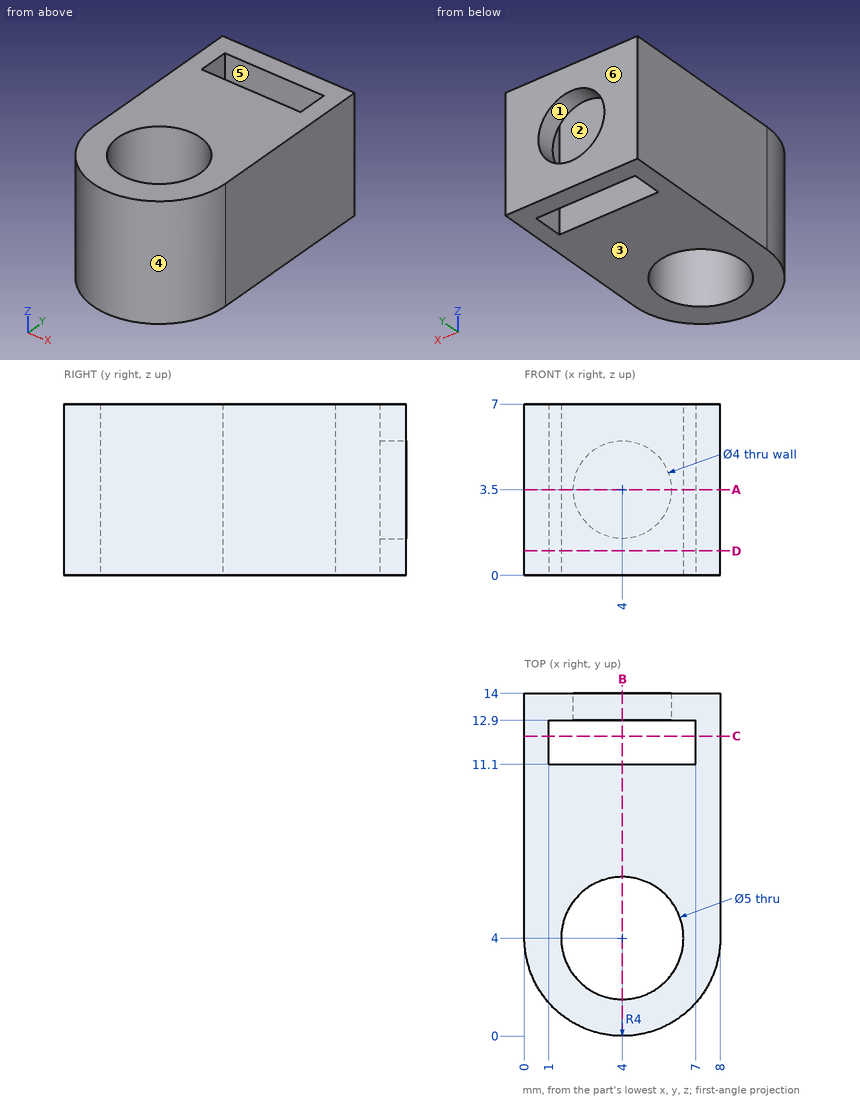
Verification items for this drawing (mm, ordinates from the low corner). A direction names the side the tool comes from. Round coordinates to 2 decimals unless told otherwise and drop trailing zeros. Order: outer loops, then holes, each group sorted by start corner. A loop starts at its lowest first (then second) coordinate and runs counter-clockwise, first axis right, second up. Notation, with made-up numbers: (-1.5, -19) - (10.5, -19) arc R19 cw to (10.5, 9) - close; hole circle Ø9 at (-26.5, -21.5). An arc over 180 degrees is marked (long way). Use CSV: the item, a comma, the result in double quotes. Start each with the question number.
1) Section check B-B, the plane x = 4. Record the cut outline in (y, z), plus the area to 3 significant figures.
2) Go/stop test with a flat-tipped pin: P1, Ø4.5, axis at x = 4, y = 4, coming from the +Z side. Record where the tip stops, or that it passes through.
3) Access from +Z, -Z, +X, -X, +Y, -Y to the whole of each face (thin tool, end or side, straight path). Record for the marked faces 1, 2 and 3.
4) Section check D-D, the plane z = 1. Record the cut outline in (x, y), plus the area to 3 significant figures.
5) Section check A-A, the plane z = 3.5. Record the cut outline in (x, y), plus the area to 3 significant figures.
6) Thickness scan on L1, parallel to X at y = 13.6, z = 3.5; L2, parallel to X at y = 11.5, z = 3; L3, parallel to Y at x = 2, z = 2.5. Record the ranges inside material, lowest first.
7) Section check C-C, the plane y = 12.25. Record the cut outline in (x, z), plus the area to 3 significant figures.
8) Mould release check, pull along Y, two halves, no side actions. Record for the marked faces 4, 5 and 6: +Y half, -Y half, draft (parallel to the pull), parting line (faces both ways), or undercut.
Answers:
1,outline,"(0, 0) - (1.5, 0) - (1.5, 7) - (0, 7) - close; (6.5, 0) - (11.1, 0) - (11.1, 7) - (6.5, 7) - close; (12.9, 0) - (14, 0) - (14, 1.5) - (12.9, 1.5) - close; (12.9, 5.5) - (14, 5.5) - (14, 7) - (12.9, 7) - close"
1,area,"46.0 mm²"
2,P1,"passes through"
3,face 1,"+Y"
3,face 2,"+Z, -Z"
3,face 3,"-Z, +X, -X, +Y, -Y"
4,outline,"(0, 4) arc R4 ccw to (8, 4) - (8, 14) - (0, 14) - close; hole (1, 11.1) - (7, 11.1) - (7, 12.9) - (1, 12.9) - close; hole circle Ø5 at (4, 4)"
4,area,"74.7 mm²"
5,outline,"(0, 4) arc R4 ccw to (8, 4) - (8, 14) - (6, 14) - (6, 12.9) - (7, 12.9) - (7, 11.1) - (1, 11.1) - (1, 12.9) - (2, 12.9) - (2, 14) - (0, 14) - close; hole circle Ø5 at (4, 4)"
5,area,"70.3 mm²"
6,L1,"x = 0 to 2, 6 to 8"
6,L2,"x = 0 to 1, 7 to 8"
6,L3,"y = 0.54 to 2.5, 5.5 to 11.1, 12.9 to 14"
7,outline,"(0, 0) - (1, 0) - (1, 7) - (0, 7) - close; (7, 0) - (8, 0) - (8, 7) - (7, 7) - close"
7,area,"14.0 mm²"
8,face 4,"-Y half"
8,face 5,"undercut"
8,face 6,"+Y half"
